```python
from build123d import *

# Parameters (mm, degrees)
F0_R     = 41.063309
F1_DEPTH = 43.841228
F2_R     = 9.936428
F4_R     = 23.134928
F5_DEPTH = 27.268376
F6_D     = 50.8


with BuildPart() as f1:
    # F0 (on Front) → F1 (new body)
    with BuildSketch(Plane.XZ):
        Circle(F0_R)
    extrude(amount=F1_DEPTH)

    # F2
    f2_edges = [f1.edges().sort_by_distance(p)[0] for p in [
        (-41.063309, -43.841228, 0),
        (41.063309, -21.920614, 0),
        (-41.063309, 0, 0),
    ]]
    fillet(f2_edges, radius=F2_R)

    # F4 (on face) → F5 (join)
    with BuildSketch(Plane.XZ.offset(43.841228)):
        Circle(F4_R)
    extrude(amount=-F5_DEPTH)

    # F6 (through all)
    with Locations(Plane.XZ.offset(43.841228)):
        with Locations((0, 0)):
            Hole(F6_D / 2)


solid = f1.part
```
Check sheet for the modelled part. Datum: model origin and axes. Units: mm. Round coordinates to 2 decimals unless told otherwise and drop trailing zeros. Order: outer loops, then holes, each group sorted by start corner. A loop starts at its lowest first (then second) coordinate and runs counter-clockwise, first axis right, second up. Notation, with made-up numbers: (46.5, -24.75) -> (90.5, -24.75) arc R28 ccw to (90.5, 0.25) -> close; hole circle Ø4 at (66, -34). An arc over 180 degrees is marked (long way). Use CSV: the item, a comma, the result in double quotes.
(1) Cross-section at A-A (x = 0). Record the boundary of the cut face in (y, z).
Worked out:
outline,"(-43.84, -31.13) arc R9.94 ccw to (-33.9, -41.06) -> (-9.94, -41.06) arc R9.94 ccw to (0, -31.13) -> (0, -25.4) -> (-43.84, -25.4) -> close; (-43.84, 25.4) -> (0, 25.4) -> (0, 31.13) arc R9.94 ccw to (-9.94, 41.06) -> (-33.9, 41.06) arc R9.94 ccw to (-43.84, 31.13) -> close"
(2) Cross-section at B-B (z = 0). Record the boundary of the cut face in (x, y), and give its area (3 significant figures).
Worked out:
outline,"(-41.06, -33.9) arc R9.94 ccw to (-31.13, -43.84) -> (-25.4, -43.84) -> (-25.4, 0) -> (-31.13, 0) arc R9.94 ccw to (-41.06, -9.94) -> close; (25.4, -43.84) -> (31.13, -43.84) arc R9.94 ccw to (41.06, -33.9) -> (41.06, -9.94) arc R9.94 ccw to (31.13, 0) -> (25.4, 0) -> close"
area,"1,290 mm²"
(3) Depth check by flat-ended pin: pin 1 (2 mm diameter, centred on x = 22, y = -10, fed in from +Z); pin 2 (5 mm diameter, centred on x = 29.5, z = -27.5, fed in from -Y); pin 3 (1 mm diameter, centred on x = -30.5, y = -30.5, fed in from +Z). Enter the tip coordinate at first touch or a pass-through.
Worked out:
pin 1,"z = 35.29"
pin 2,"y = -41.24"
pin 3,"z = 28.04"
(4) Cross-section at D-D (y = -38). Record the boundary of the cut face in (x, z).
Worked out:
outline,"circle Ø80.36 at (0, 0); hole circle Ø50.8 at (0, 0)"
(5) Material ranges on line 1 along Z through (x, y) = (0, -15); line 2 along X through (y, z) = (-40, -10); line 3 along X through (y, z) = (-34, 5), recorded low to high. Write a range as from..to.
Worked out:
line 1,"-41.06..-25.4, 25.4..41.06"
line 2,"-37.67..-23.35, 23.35..37.67"
line 3,"-40.76..-24.9, 24.9..40.76"
(6) Cross-section at C-C (y = -32). Record the boundary of the cut face in (x, z).
Worked out:
outline,"circle Ø82.13 at (0, 0); hole circle Ø50.8 at (0, 0)"
(7) Draft check along Z on faces 1 (the face through (-5.346, -21.753, 40.714)), 2 (the face through (5.506, -21.614, -24.796)), 3 (the face through (-26, -43.841, 0)). Enter one of: pulls with the +Z half, pulls with the -Z half, needs draft (parallel to the pull), parting line crosses it, or undercut.
Worked out:
face 1,"parting line crosses it"
face 2,"undercut"
face 3,"needs draft"
